Geometry: final body of the model. Coordinates: model frame, mm. A direction names the side the tool comes from. Coordinates: 2 decimals unless noted, no trailing zeros. Order: outer loops, then holes, each group sorted by start corner. A loop starts at its lowest first (then second) coordinate and runs counter-clockwise, first axis right, second up. Notation, with made-up numbers: M 42,14.25 L 99,14.25 A15 ccw 99,42.25 Z; hole C 82,20 d8. An arc over 180 degrees is marked long. Use CSV: the item, a comma, the result in double quotes. Start each with the question number.
Q1. Section query D-D, the plane z = -7. Output: boundary loops of the cut face in (x, y) (3 decimals), and give its area (3 significant figures).
Q2. Mould query, pull axis Y, two halves, no side actions, for faces 1 (the face through (79.375, -58, 0)), 2 (the face through (-1, -95.25, 0)), 3 (the face through (-37, -94, 25.4)). Classes: +Y half, -Y half, draft (parallel to the pull), parting line (faces both ways), or undercut.
Q3. Ray query, probe 1 along Y at (x, z) = (-4, -4) (3 decimals); probe 2 along Y at (x, z) = (72, 10.5) (3 decimals); probe 3 along Z at (x, y) = (-9.5, 68.5). Return the intervals inside material, ascending.
Q4. Access query for faces 4 (the face through (82.55, -48, 0)), 5 (the face through (-1, -92.075, 0)). Directions: +Z, -Z, +X, -X, +Y, -Y. A direction counts if a zero-diameter tool reaches every point of the face in a straight line with its end or side. Return the directions, or none.
Q5. Section query B-B, the plane x = -23.5. Output: boundary loops of the cut face in (y, z) (3 decimals), and give its area (3 significant figures).
Q6. Section query C-C, the plane y = -42.5. Output: boundary loops of the cut face in (x, z) (3 decimals).
Q7. First-contact query: P1, Ø8, axis at y = -73, z = 33.5, coming from the -X side; P2, Ø4, axis at y = 46, z = 0.5, coming from the -X side; P3, Ø3, axis at x = -27.5, y = 11.5, coming from the +Z side; P4, Ø14.5, axis at x = 0, y = 0, coming from the +Z side. Flat tips, straight axial feed; report the tip coordinate or a pass-through.
Q8. Section query A-A, the plane x = 0. Output: boundary loops of the cut face in (y, z) (3 decimals).
from build123d import *

# Parameters (mm, degrees)
CUT_EXTRUDE1_DEPTH       = 140.411064841
CUT_EXTRUDE1_DEPTH_BACK  = 140.411064841
SKETCH2_R                = 6.35
SKETCH3_W                = 165.1
SKETCH3_H                = 50.8
BOSS_EXTRUDE1_DEPTH      = 3.175
BOSS_EXTRUDE2_REACH      = 209.561
BOSS_EXTRUDE2_END_RADIUS = 82.55
SKETCH5_W                = 3.175
SKETCH5_H                = 50.8


with BuildPart() as part:
    # Sketch1 → Revolve1 (revolve)
    with BuildSketch(Plane(origin=(0, 0, 0), x_dir=(0, 0, -1), z_dir=(1, 0, 0)), mode=Mode.PRIVATE) as revolve1_sk:
        with BuildLine():
            Line((25.4, 82.55), (-25.4, 82.55))
            ThreePointArc((-25.4, 82.55), (-62.482566405, 48.464271634), (-76.2, 0))
            Line((-76.2, 0), (76.2, 0))
            ThreePointArc((76.2, 0), (62.482566405, 48.464271634), (25.4, 82.55))
        make_face()
    revolve(revolve1_sk.sketch.rotate(Axis((0, 0, -76.2), (0, 0, 1)), 90), axis=Axis((0, 0, -76.2), (0, 0, 1)))

    # Sketch2 → Cut-Extrude1 (cut, two sides: drawn at the far end of the back side and taken through both)
    with BuildSketch(Plane.XY.offset(-CUT_EXTRUDE1_DEPTH_BACK)):
        with Locations(Location((0, 0, 0), (0, 0, 90))):
            Circle(SKETCH2_R)
    extrude(amount=CUT_EXTRUDE1_DEPTH + CUT_EXTRUDE1_DEPTH_BACK, mode=Mode.SUBTRACT)



with BuildPart() as body_2:
    # Sketch3 → Boss-Extrude1 (new body)
    with BuildSketch(Plane(origin=(0, -95.25, 0), x_dir=(1, 0, 0), z_dir=(0, 1, 0))):
        Rectangle(SKETCH3_W, SKETCH3_H)
    extrude(amount=BOSS_EXTRUDE1_DEPTH)


with BuildPart() as part_1:
    add(part.part)

    add(body_2.part)  # Boss-Extrude2 merges body 2
    # Boss-Extrude2: up to this cylinder (the profile starts outside it)
    boss_extrude2_end = Plane(origin=(0, 0, 0), z_dir=(0, 0, -1)) * Cylinder(BOSS_EXTRUDE2_END_RADIUS, 585.222, mode=Mode.PRIVATE)
    # Sketch5 → Boss-Extrude2 (add, up to the surface)
    with BuildSketch(Plane(origin=(0, -92.075, 0), x_dir=(1, 0, 0), z_dir=(0, 1, 0)), mode=Mode.PRIVATE) as boss_extrude2_sk1:
        with Locations((80.9625, 0)):
            Rectangle(SKETCH5_W, SKETCH5_H)
    boss_extrude2_tool1 = extrude(boss_extrude2_sk1.sketch, amount=BOSS_EXTRUDE2_REACH, mode=Mode.PRIVATE) - boss_extrude2_end
    add(boss_extrude2_tool1.solids().sort_by_distance((80.9625, -92.075, 0))[0])
    # Sketch5 → Boss-Extrude2 (add, up to the surface)
    with BuildSketch(Plane(origin=(0, -92.075, 0), x_dir=(1, 0, 0), z_dir=(0, 1, 0)), mode=Mode.PRIVATE) as boss_extrude2_sk2:
        with Locations((-80.9625, 0)):
            Rectangle(SKETCH5_W, SKETCH5_H)
    boss_extrude2_tool2 = extrude(boss_extrude2_sk2.sketch, amount=BOSS_EXTRUDE2_REACH, mode=Mode.PRIVATE) - boss_extrude2_end
    add(boss_extrude2_tool2.solids().sort_by_distance((-80.9625, -92.075, 0))[0])


solid = part_1.part
Responses:
1,outline,"M -82.55,-95.25 L 82.55,-95.25 L 82.55,0 A82.55 ccw -82.55,0 Z; hole M -79.375,-92.075 L 79.375,-92.075 L 79.375,-22.674 A82.55 cw -79.375,-22.674 Z; hole C 0,0 d12.7"
1,area,"22,300 mm²"
2,face 1,"undercut"
2,face 2,"-Y half"
2,face 3,"draft"
3,probe 1,"y = -95.25 to -92.075, -82.453 to -4.932, 4.932 to 82.453"
3,probe 2,"y = -95.25 to -92.075, -40.379 to 40.379"
3,probe 3,"z = -45.12 to 45.12"
4,face 4,"+Z, -Z, +X, +Y, -Y"
4,face 5,"+Z, -Z"
5,outline,"M -95.25,-25.4 L -92.075,-25.4 L -92.075,25.4 L -95.25,25.4 Z; M -79.134,-25.4 A89.436 ccw 79.134,-25.4 L 79.134,25.4 A89.436 ccw -79.134,25.4 Z"
5,area,"19,000 mm²"
6,outline,"M -82.55,-25.4 L -79.375,-25.4 L -79.375,25.4 L -82.55,25.4 Z; M -70.769,-25.4 A82.127 ccw 70.769,-25.4 L 70.769,25.4 A82.127 ccw -70.769,25.4 Z; M 79.375,-25.4 L 82.55,-25.4 L 82.55,25.4 L 79.375,25.4 Z"
7,P1,"stops at x = -37.89"
7,P2,"stops at x = -69.85"
7,P3,"stops at z = 71.76"
7,P4,"stops at z = 75.98"
8,outline,"M -95.25,-25.4 L -92.075,-25.4 L -92.075,25.4 L -95.25,25.4 Z; M -82.55,-25.4 A92.472 ccw -6.35,-75.982 L -6.35,75.982 A92.472 ccw -82.55,25.4 Z; M 6.35,-75.982 A92.472 ccw 82.55,-25.4 L 82.55,25.4 A92.472 ccw 6.35,75.982 Z"
